Check sheet for the modelled part. Datum: model origin and axes. Units: mm. Face numbers are marked on the shaded views. A direction names the side the tool comes from. Round coordinates to 2 decimals unless told otherwise and drop trailing zeros. Write each loop counter-clockwise with the first axis right and the second up, starting at its lowest first coordinate (ties: lowest second). Pieces come first, ordered by that corner, then holes.
Item 1: Section check B-B, the plane z = 8.5. Record the cut outline in (x, y), plus the area to 3 significant figures.
Item 2: Section check D-D, the plane y = -46. Record the cut outline in (x, z).
Item 3: Depth check by flat-ended pin: pin 1 (3 mm diameter, centred on x = -2.5, z = 6.5, fed in from -Y). Enter the tip coordinate at first touch or a pass-through.
Item 4: Set-up check for the marked faces 1 and 2: record each of +Z, -Z, +X, -X, +Y, -Y from which the full face is reachable in a straight line by a thin tool's end or side.
Item 5: Section check C-C, the plane y = -40. Record the cut outline in (x, z), plus the area to 3 significant figures.
Item 6: Section check A-A, the plane x = -10. Record the cut outline in (y, z).
Item 7: Material ranges on line 1 along X through (y, z) = (-35.5, 10); line 2 along Y through (x, z) = (2.5, 6.5); line 3 along Z through (x, y) = (1, -43.25), recorded low to high.
from build123d import *

# Parameters (mm, degrees)
F0_W     = 30
F0_H     = 15
F1_DEPTH = 15
F2_W     = 15
F2_H     = 15
F3_DEPTH = 5
F4_W     = 10
F4_H     = 4.995112
F5_DEPTH = 15
F7_DEPTH = 15


with BuildPart() as f1:
    # F0 (on Top) → F1 (new body)
    with BuildSketch(Plane.XY):
        with Locations((-11.458107, -42.121633)):
            Rectangle(F0_W, F0_H)
    extrude(amount=F1_DEPTH)

    # F2 (on face) → F3 (cut)
    with BuildSketch(Plane.XZ.offset(49.621633)):
        with Locations((-3.958107, 7.5)):
            Rectangle(F2_W, F2_H)
    extrude(amount=-F3_DEPTH, mode=Mode.SUBTRACT)

    # F4 (on face) → F5 (cut)
    with BuildSketch(Plane.YZ.offset(3.541893)):
        with Locations((-39.621633, 12.502444)):
            Rectangle(F4_W, F4_H)
    extrude(amount=-F5_DEPTH, mode=Mode.SUBTRACT)

    # F6 (on face) → F7 (cut)
    with BuildSketch(Plane.YZ.offset(3.541893)):
        Polygon((-44.621633, 10.004888), (-44.621633, 0), (-34.621633, 10.004888), align=None)
    extrude(amount=-F7_DEPTH, mode=Mode.SUBTRACT)


solid = f1.part
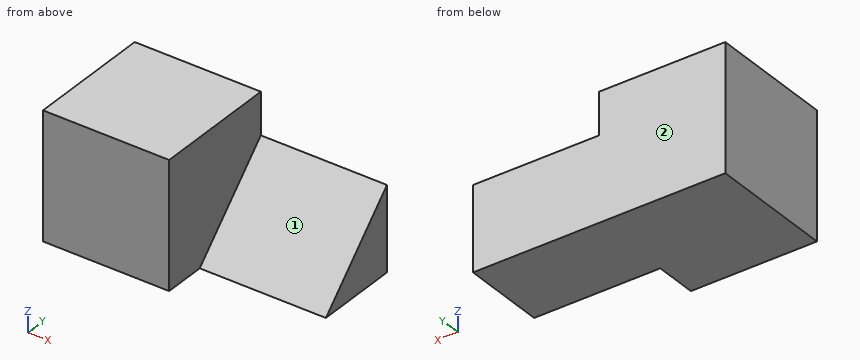
Values found:
1. outline: (-26.46, -49.62) - (-11.46, -49.62) - (-11.46, -36.13) - (3.54, -36.13) - (3.54, -34.62) - (-26.46, -34.62) - close
1. area: 248 mm2
2. outline: (-26.46, 0) - (-11.46, 0) - (-11.46, 15) - (-26.46, 15) - close
3. pin 1: stops at y = -39.62
4. face 1: +Z, +X, -Y
4. face 2: +Z, -Z, +X, -X, +Y
5. outline: (-26.46, 0) - (3.54, 0) - (3.54, 4.62) - (-11.46, 4.62) - (-11.46, 15) - (-26.46, 15) - close
5. area: 294 mm2
6. outline: (-44.62, 0) - (-34.62, 0) - (-34.62, 10) - close
7. line 1: x = -26.46 to -11.46
7. line 2: y = -38.12 to -34.62
7. line 3: z = 0 to 1.37
